The model under review builds one solid part; all positions refer to its coordinate system, in mm. A direction names the side the tool comes from. Give positions to 0.01 mm unless a question says otherwise; leave off trailing zeros. Order: outer loops, then holes, each group sorted by start corner. A loop starts at its lowest first (then second) coordinate and runs counter-clockwise, first axis right, second up. Notation, with made-up numbers: (69.25, 89) - (127.25, 89) arc R12 ccw to (127.25, 109) - close; hole circle Ø8 at (51.5, 55.25). An arc over 180 degrees is marked (long way). Put each result on its own line as item: value.
Autodesk Inventor part; units mm, degrees
ref_plane "YZ Plane" through (0, 0, 0) normal (1, 0, 0) x (0, 1, 0)
ref_plane "XZ Plane" through (0, 0, 0) normal (0, 1, 0) x (-1, 0, 0)
ref_plane "XY Plane" through (0, 0, 0) normal (0, 0, 1) x (1, 0, 0)
sketch "Szkic1" plane through (0, 0, 0) normal (0, 1, 0) x (-1, 0, 0)
  line L0 (-50, -50) -> (50, -50)
  line L1 (50, -50) -> (50, 50)
  line L2 (50, 50) -> (-50, 50)
  line L3 (-50, 50) -> (-50, -50)
  line L4 (-50, -50) -> (50, 50) construction
  line L5 (50, -50) -> (-50, 50) construction
  point P0 (0, 0)
  dimension "d0" = 100
  dimension "d1" = 100
extrude "Wyciągnięcie proste1" add sketch "Szkic1" along normal blind 20
sketch "Szkic2" plane through (0, 20, 0) normal (0, 1, 0) x (1, 0, 0)
  line L0 (-48, 48) -> (48, 48)
  line L1 (48, 48) -> (48, -48)
  line L2 (48, -48) -> (-48, -48)
  line L3 (-48, -48) -> (-48, 48)
  line L4 (-48, 48) -> (48, -48) construction
  line L5 (48, 48) -> (-48, -48) construction
  point P0 (0, 0)
  dimension "d4" = 96
  dimension "d5" = 96
extrude "Wyciągnięcie proste2" cut sketch "Szkic2" against normal blind 10
fillet "Zaokrąglenie1" radius 4 8 edges at (-48, 15, 48) (-50, 10, 50) (-50, 10, -50) (-48, 15, -48) (50, 10, -50) (48, 15, -48) (50, 10, 50) (48, 15, 48)
equation "\"PromieńGięcia\" = Grubość"
equation "\"SzerokośćGięciaPodcięcia\" = Grubość"
equation "\"GłębokośćGięciaPodcięcia\" = 0.5 * Grubość"
equation "\"RozmiarPodcięciaNarożnika\" = 4 * Grubość"
equation "\"MinimalnaPozostałość\" = 2 * Grubość"
equation "\"PromieńPrzejścia\" = PromieńGięcia"
equation "\"Rozmiar_promienia_Jacobiego\" = PromieńGięcia"
equation "\"Wielk_odstępu\" = Grubość"
(1) The part is to be moulded in two halves that separate along Z. For faces 3 (the flat face through (-50, 10, -1)), 4 (the cylindrical face through (-46.797, 14.93, 46.859)), 5 (the flat face through (-1, 10, 50)), say which applies: pulls with the +Z half, pulls with the -Z half, needs draft (parallel to the pull), parting line crosses it, or undercut.
The answers:
face 3: needs draft
face 4: undercut
face 5: pulls with the +Z half
(2) For faces 1 (the cylindrical face through (-48.797, 10.14, -48.859)), 2 (the flat face through (48, 15, -1)), list the 3-axis set-ups (+Z, -Z, +X, -X, +Y, -Y) from which the entire face can be reached by the end or side of a thin tool; tool diameter is ignored.
The answers:
face 1: -Z, -X, +Y, -Y
face 2: +Y
(3) Clearance check with a flat-ended pin moving along its axis: pin 1 Ø1.5 at (x, z) = (33, 9) entering from +Y. State where the tip first meets the part, or that it passes through.
The answers:
pin 1: y = 10
(4) Take a section at A-A, the plane y = 14.5. Write out the cut boundary in (x, z), then the cut area to 3 significant figures.
The answers:
outline: (-50, -46) arc R4 ccw to (-46, -50) - (46, -50) arc R4 ccw to (50, -46) - (50, 46) arc R4 ccw to (46, 50) - (-46, 50) arc R4 ccw to (-50, 46) - close; hole (-48, -44) arc R4 ccw to (-44, -48) - (44, -48) arc R4 ccw to (48, -44) - (48, 44) arc R4 ccw to (44, 48) - (-44, 48) arc R4 ccw to (-48, 44) - close
area: 784 mm^2
(5) Take a section at C-C, the plane z = 7.5. Write out the cut boundary in (x, y).
The answers:
outline: (-50, 0) - (50, 0) - (50, 20) - (48, 20) - (48, 10) - (-48, 10) - (-48, 20) - (-50, 20) - close
(6) Wall thickness on L1, parallel to X at y = 18.25, z = 21.5; L2, parallel to Y at x = -17, z = -24: over which ranges is each line inside the solid? List them lowest first.
The answers:
L1: -50 to -48, 48 to 50
L2: 0 to 10
(7) Take a section at B-B, the plane x = 14.5. Write out the cut boundary in (y, z), then the cut area to 3 significant figures.
The answers:
outline: (0, -50) - (20, -50) - (20, -48) - (10, -48) - (10, 48) - (20, 48) - (20, 50) - (0, 50) - close
area: 1,040 mm^2
